Can you work these out from the model? Positions are in its coordinate system, mm. Give positions to 0.01 mm unless a question says otherwise; leave off trailing zeros. Write each loop counter-clockwise with the first axis right and the second up, starting at its lowest first coordinate (ties: lowest second). Pieces come first, ordered by that corner, then holes.
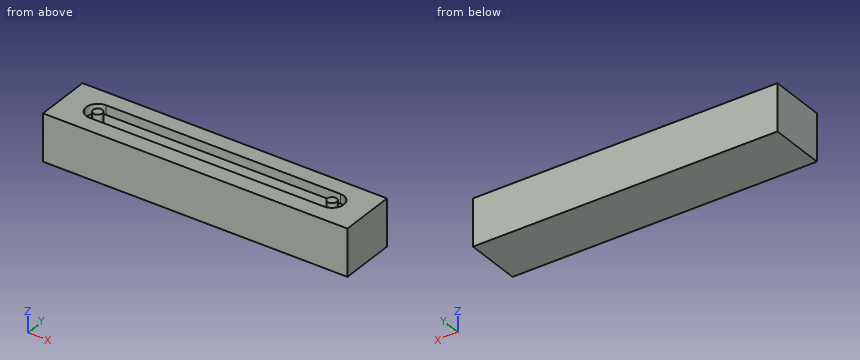
Autodesk Fusion 360 part; units mm, degrees
sketch "Sketch1" plane through (0, 0, 0) normal (0, 0, 1) x (1, 0, 0)
  line L0 (0, 0) -> (-55, 0)
  line L1 (-55, 0) -> (-55, -12)
  line L2 (-55, -12) -> (0, -12)
  line L3 (0, -12) -> (0, 0)
  dimension "d1" = 12
  dimension "d2" = 55
extrude "Extrude1" add sketch "Sketch1" along normal blind 10
sketch "Sketch2" plane through (0, 0, 10) normal (0, 0, 1) x (-1, 0, 0)
  line L0 (0, 12) -> (0, 0)
  line L1 (0, 0) -> (55, 0)
  line L2 (55, 0) -> (55, 12)
  line L3 (55, 12) -> (0, 12)
  line L4 (0, 6) -> (55, 6)
  line L5 (27.5, 12) -> (27.5, 0)
  line L6 (27.5, 6) -> (2.5, 6)
  line L7 (27.5, 6) -> (52.5, 6)
  circle A0 centre (2.5, 6) radius 1
  circle A1 centre (2.5, 6) radius 2.5
  circle A2 centre (52.5, 6) radius 1
  circle A3 centre (52.5, 6) radius 2.5
  line L8 (2.5, 6) -> (2.5, 3.5)
  line L9 (52.5, 3.5) -> (2.5, 3.5)
  line L10 (2.5, 8.5) -> (52.5, 8.5)
  dimension "d5" = 25
  dimension "d6" = 25
  dimension "d7" = 2
  dimension "d8" = 5
  dimension "d9" = 2
  dimension "d10" = 5
extrude "Extrude2" add 1 faces at (0, -8, 3.3333) along direction (1, 0, 0) blind 5
extrude "Extrude3" add 1 faces at (-55, -4, 3.3333) along direction (-1, 0, 0) blind 5
extrude "Extrude4" cut sketch "Sketch2" against normal blind 2 contours L4 L6 A0 A1 | L4 A0 A1 L8 | L4 L5 L6 A1 L10 | L4 L6 A0 A1 L8 | L4 L5 L6 A1 L9 | L4 L5 L7 A3 L10 | L4 L5 L7 A3 L9 | L4 L7 A2 A3 | L4 L7 A2 A3
(1) Imagine slicing it at C-C, the plane x = -48.5. Write out the boundary of the cut face in (y, z).
Returned:
outline: (-12, 0) - (0, 0) - (0, 10) - (-3.5, 10) - (-3.5, 8) - (-8.5, 8) - (-8.5, 10) - (-12, 10) - close
(2) Imagine slicing it at B-B, the plane y = -6. Write out the boundary of the cut face in (x, z).
Returned:
outline: (-60, 0) - (5, 0) - (5, 10) - (0, 10) - (0, 8) - (-1.5, 8) - (-1.5, 10) - (-3.5, 10) - (-3.5, 8) - (-51.5, 8) - (-51.5, 10) - (-53.5, 10) - (-53.5, 8) - (-55, 8) - (-55, 10) - (-60, 10) - close
(3) If I drill on L1, parallel to Y at x = -42.5, z = 9.5; L2, parallel to Z at x = -6, y = -5, over which ranges is the centre line in solid material (lowest first)?
Returned:
L1: y = -12 to -8.5, -3.5 to 0
L2: z = 0 to 8
(4) Imagine slicing it at A-A, the plane z = 9.25. Write out the boundary of the cut face in (x, y), plus the area to 3 significant figures.
Returned:
outline: (-60, -12) - (5, -12) - (5, 0) - (-60, 0) - close; circle Ø2 at (-52.5, -6); circle Ø2 at (-2.5, -6); hole (-52.5, -8.5) - (-2.5, -8.5) arc R2.5 ccw to (-2.5, -3.5) - (-52.5, -3.5) arc R2.5 ccw to start
area: 517 mm2
